Check sheet for the modelled part. Datum: model origin and axes. Units: mm. A direction names the side the tool comes from. Give positions to 0.01 mm unless a question says otherwise; leave off trailing zeros. Order: outer loops, then holes, each group sorted by start corner. A loop starts at its lowest first (then second) coordinate and runs counter-clockwise, first axis right, second up.
Autodesk Inventor part; units mm, degrees
ref_plane "YZ Plane" through (0, 0, 0) normal (1, 0, 0) x (0, 1, 0)
ref_plane "XZ Plane" through (0, 0, 0) normal (0, 1, 0) x (-1, 0, 0)
ref_plane "XY Plane" through (0, 0, 0) normal (0, 0, 1) x (1, 0, 0)
sketch "Boceto1" plane through (0, 0, 0) normal (0, 1, 0) x (-1, 0, 0)
  line L0 (0, 0) -> (180, 0)
  line L1 (180, 0) -> (180, -240)
  line L2 (180, -240) -> (0, -240)
  line L3 (0, -240) -> (0, 0)
  line L4 (-3, -243) -> (183, -243)
  line L5 (183, -243) -> (183, 3)
  line L6 (183, 3) -> (-3, 3)
  line L7 (-3, 3) -> (-3, -243)
  line L8 (203, 23) -> (203, -263)
  line L9 (203, -263) -> (-23, -263)
  line L10 (-23, -263) -> (-23, 23)
  line L11 (-23, 23) -> (203, 23)
  dimension "d0" = 180
  dimension "d1" = 240
  dimension "d2" = 3
  dimension "d5" = 20
extrude "Extrusión2" add sketch "Boceto1" along normal blind 30 contours L7 L6 L5 L4
extrude "Extrusión3" add sketch "Boceto1" along normal blind 3 contours L8 L9 L10 L11
fillet "Empalme1" radius 2 4 edges at (3, 3, -120) (-90, 3, 3) (-90, 3, -243) (-183, 3, -120)
sketch "Boceto3" plane through (0, 3, 0) normal (0, 1, 0) x (1, 0, 0)
  line L0 (23, -23) -> (23, 263)
  line L1 (23, 263) -> (-203, 263)
  line L2 (-203, 263) -> (-203, -23)
  line L3 (-203, -23) -> (23, -23)
  line L4 (-185, -5) -> (5, -5)
  line L5 (-185, 245) -> (-185, -5)
  line L6 (5, 245) -> (-185, 245)
  line L7 (5, -5) -> (5, 245)
  line L8 (-203, 263) -> (-203, -23)
  line L9 (-203, -23) -> (-203, 2)
  line L10 (-185, 245) -> (-185, -5)
  line L11 (-203, 2) -> (-185, 2)
  line L12 (-185, 2) -> (-185, 52)
  line L13 (-185, 52) -> (-203, 52)
  line L14 (-203, 52) -> (-203, 2)
  line L15 (-183, 243) -> (-183, -3)
  line L16 (-203, 182) -> (-183, 182)
  line L17 (-183, 182) -> (-183, 232)
  line L18 (-183, 232) -> (-203, 232)
  line L19 (-203, 232) -> (-203, 182)
  line L20 (5, -5) -> (5, 245)
  line L21 (23, 207) -> (23, 232)
  line L22 (5, 232) -> (5, 207)
  circle A0 centre (14, 188) radius 3.175
  circle A1 centre (14, 52) radius 3.1767
  point P0 (0, 0)
  point P1 (-193, 182)
  point P2 (-185, 232)
  point P3 (-185, 182)
  dimension "d11" = 25
  dimension "d12" = 50
  dimension "d13" = 50
  dimension "d14" = 130
  dimension "d15" = 6.35
  dimension "d16" = 75
  dimension "d17" = 75
extrude "Extrusión5" cut sketch "Boceto3" against normal blind 3 contours A0 | A1
properties part number "Tapa Superior"
(1) Sectioned sample at C-C (y = 11.75). Enter the section's corners in (x, z).
(2) Thickness scan on L1, parallel to X at y = 0.9, z = -188 (3 decimals); L2, parallel to Z at x = 14, y = 1 (3 decimals); L3, parallel to X at y = 5.5, z = -140. Record the ranges inside material, lowest first.
(3) Tool access check on faces 1 (the face through (-89, 15, 0)), 2 (the face through (3, 17, -118)), 3 (the face through (-183, 17, -122)), 4 (the face through (-189, 3, -118)). Record the directions out of +Z, -Z, +X, -X, +Y, -Y that give a thin tool (end or side, any length) a straight path to the whole face; none if there is none.
(4) Sectioned sample at A-A (x = 14). Enter the section's corners in (y, z) (3 decimals), plus the area to 3 significant figures.
(5) Go/stop test with flat-tipped pins: P1, Ø1.5, axis at y = 8, z = -228, coming from the +X side; P2, Ø7.5, axis at x = 14, z = -188, coming from the +Y side; P3, Ø2, axis at x = -66.5, y = 25, coming from the +Z side; P4, Ø12, axis at x = -72, z = -230, coming from the -Y side. Record where each tip stops, or that it passes through.
(6) Release check for a two-part mould opening along Z. For faces 5 (the face through (-89, 17, -243)), 6 (the face through (0, 15, -122)), 7 (the face through (-189, 0, -118)) record: released by +Z, released by -Z, zero draft, split by the parting line, or undercut.
(7) Sectioned sample at B-B (z = -153). Enter the section's corners in (x, y), plus the area to 3 significant figures.
(8) Sectioned sample at D-D (x = -12). Enter the section's corners in (y, z).
Values follow:
1. outline: (-183, -243) - (3, -243) - (3, 3) - (-183, 3) - close; hole (-180, -240) - (0, -240) - (0, 0) - (-180, 0) - close
2. L1: x = -203 to -180, 0 to 10.825, 17.175 to 23
2. L2: z = -263 to -191.175, -184.825 to -55.177, -48.823 to 23
2. L3: x = -183 to -180, 0 to 3
3. face 1: +Y, -Y
3. face 2: +Z, -Z, +X, +Y
3. face 3: +Z, -Z, -X, +Y
3. face 4: +Y
4. outline: (0, -263) - (3, -263) - (3, -191.175) - (0, -191.175) - close; (0, -184.825) - (3, -184.825) - (3, -55.177) - (0, -55.177) - close; (0, -48.823) - (3, -48.823) - (3, 23) - (0, 23) - close
4. area: 820 mm2
5. P1: stops at x = 3
5. P2: stops at y = 3
5. P3: stops at z = 3
5. P4: passes through
6. face 5: released by -Z
6. face 6: undercut
6. face 7: zero draft
7. outline: (-203, 0) - (-180, 0) - (-180, 30) - (-183, 30) - (-183, 5) arc R2 cw to (-185, 3) - (-203, 3) - close; (0, 0) - (23, 0) - (23, 3) - (5, 3) arc R2 cw to (3, 5) - (3, 30) - (0, 30) - close
7. area: 302 mm2
8. outline: (0, -263) - (3, -263) - (3, -245) arc R2 cw to (5, -243) - (30, -243) - (30, -240) - (0, -240) - close; (0, 0) - (30, 0) - (30, 3) - (5, 3) arc R2 cw to (3, 5) - (3, 23) - (0, 23) - close
